The listing builds one solid part. Answer for the finished solid, in the listing's coordinates (mm). Round coordinates to 2 decimals unless told otherwise and drop trailing zeros. Write each loop counter-clockwise with the first axis right and the second up, starting at its lowest first coordinate (ties: lowest second). Pieces come first, ordered by that corner, then holes. Notation, with made-up numbers: (79, 47.5) - (85, 47.5) arc R32 ccw to (85, 75.5) - close; hole circle Ø4 at (38.5, 44). An arc over 180 degrees is marked (long way). Use a Markdown table: item, result. Add a question column.
1) A cutting plane is placed at A-A (z = 74.5). Give the vertices of the cut face in (x, y).
2) Find the intervals of material crossed by probe 1 along Z at (x, y) = (0, 2.1); probe 2 along Z at (x, y) = (60, 2.2); probe 3 along X at (y, z) = (2.15, 72), in increasing order. Write a range as from..to.
3) Each of these flat-tipped pins is pushed along its axis until it touches: P1, Ø0.9, axis at y = 1.5, z = 78, coming from the -X side; P2, Ø1.5, axis at x = 0, y = 1.5, coming from the -Z side; P3, Ø1.8, axis at x = 75, z = -60, coming from the -Y side. Where does it stop, or does it pass through?
4) A cutting plane is placed at C-C (z = 44). Give the vertices of the cut face in (x, y), then the cut area to 3 significant figures.
5) A cutting plane is placed at B-B (y = 0.95). State how many separate pieces and enclosed holes the cut face has, then the cut area to 3 significant figures.
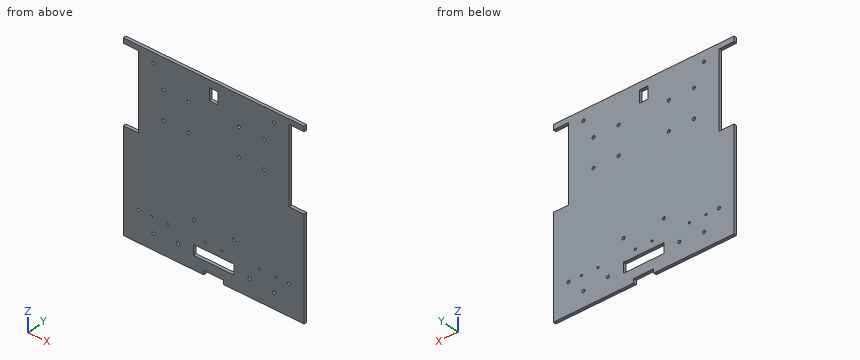
```python
from build123d import *

# Parameters (mm, degrees)
SKETCH1_W           = 180
SKETCH1_H           = 180
BOSS_EXTRUDE1_DEPTH = 3
SKETCH2_W           = 15
SKETCH2_H           = 75
CUT_EXTRUDE1_DEPTH  = 3
SKETCH3_R           = 1.5
SKETCH3_R_2         = 1
SKETCH3_W           = 40
SKETCH3_H           = 10
CUT_EXTRUDE2_DEPTH  = 3
SKETCH5_R           = 1.5
CUT_EXTRUDE3_DEPTH  = 3
SKETCH7_W           = 20
SKETCH7_H           = 4
CUT_EXTRUDE4_DEPTH  = 3
SKETCH8_W           = 8.5
SKETCH8_H           = 12
CUT_EXTRUDE5_DEPTH  = 3


with BuildPart() as part:
    # Sketch1 → Boss-Extrude1 (new body)
    with BuildSketch(Plane(origin=(0, 0, 0), x_dir=(1, 0, 0), z_dir=(0, 1, 0))):
        Rectangle(SKETCH1_W, SKETCH1_H)
    extrude(amount=BOSS_EXTRUDE1_DEPTH)

    # Sketch2 → Cut-Extrude1 (cut)
    with BuildSketch(Plane(origin=(0, 3, 0), x_dir=(1, 0, 0), z_dir=(0, 1, 0))):
        with Locations((-82.5, -47.5)):
            Rectangle(SKETCH2_W, SKETCH2_H)
        with Locations((82.5, -47.5)):
            Rectangle(SKETCH2_W, SKETCH2_H)
    extrude(amount=-CUT_EXTRUDE1_DEPTH, mode=Mode.SUBTRACT)

    # Sketch3 → Cut-Extrude2 (cut)
    with BuildSketch(Plane(origin=(0, 3, 0), x_dir=(1, 0, 0), z_dir=(0, 1, 0))):
        with Locations(Location((-50, -32.5, 0), (0, 0, 270))):
            Circle(SKETCH3_R)
        with Locations(Location((-50, -60.5, 0), (0, 0, 270))):
            Circle(SKETCH3_R)
        with Locations(Location((-25, -32.5, 0), (0, 0, 270))):
            Circle(SKETCH3_R)
        with Locations(Location((-25, -60.5, 0), (0, 0, 270))):
            Circle(SKETCH3_R)
        with Locations(Location((25, -60.5, 0), (0, 0, 90))):
            Circle(SKETCH3_R)
        with Locations(Location((50, -60.5, 0), (0, 0, 90))):
            Circle(SKETCH3_R)
        with Locations(Location((25, -32.5, 0), (0, 0, 90))):
            Circle(SKETCH3_R)
        with Locations(Location((50, -32.5, 0), (0, 0, 90))):
            Circle(SKETCH3_R)
        with Locations(Location((-60, -80, 0), (0, 0, 270))):
            Circle(SKETCH3_R)
        with Locations(Location((60, -80, 0), (0, 0, 90))):
            Circle(SKETCH3_R)
        with Locations(Location((-62, 60, 0), (0, 0, 270))):
            Circle(SKETCH3_R_2)
        with Locations(Location((-45.5, 60, 0), (0, 0, 270))):
            Circle(SKETCH3_R_2)
        with Locations(Location((45.5, 60, 0), (0, 0, 90))):
            Circle(SKETCH3_R_2)
        with Locations(Location((62, 60, 0), (0, 0, 90))):
            Circle(SKETCH3_R_2)
        with Locations(Location((-60, 75, 0), (0, 0, 270))):
            Circle(SKETCH3_R)
        with Locations(Location((60, 75, 0), (0, 0, 90))):
            Circle(SKETCH3_R)
        with Locations(Location((-8.25, 60, 0), (0, 0, 270))):
            Circle(SKETCH3_R_2)
        with Locations(Location((8.25, 60, 0), (0, 0, 90))):
            Circle(SKETCH3_R_2)
        with Locations(Location((-20, 44.727497325, 0), (0, 0, 270))):
            Circle(SKETCH3_R)
        with Locations(Location((20, 44.727497325, 0), (0, 0, 90))):
            Circle(SKETCH3_R)
        with Locations((0, 71.727497325)):
            Rectangle(SKETCH3_W, SKETCH3_H)
    extrude(amount=-CUT_EXTRUDE2_DEPTH, mode=Mode.SUBTRACT)

    # Sketch5 → Cut-Extrude3 (cut)
    with BuildSketch(Plane(origin=(0, 3, 0), x_dir=(1, 0, 0), z_dir=(0, 1, 0))):
        with Locations(Location((-75, 60, 0), (0, 0, 270))):
            Circle(SKETCH5_R)
        with Locations(Location((75, 60, 0), (0, 0, 90))):
            Circle(SKETCH5_R)
        with Locations(Location((-35.5, 73, 0), (0, 0, 270))):
            Circle(SKETCH5_R)
        with Locations(Location((35.5, 73, 0), (0, 0, 90))):
            Circle(SKETCH5_R)
    extrude(amount=-CUT_EXTRUDE3_DEPTH, mode=Mode.SUBTRACT)

    # Sketch7 → Cut-Extrude4 (cut)
    with BuildSketch(Plane(origin=(0, 3, 0), x_dir=(1, 0, 0), z_dir=(0, 1, 0))):
        with Locations((0, 88)):
            Rectangle(SKETCH7_W, SKETCH7_H)
    extrude(amount=-CUT_EXTRUDE4_DEPTH, mode=Mode.SUBTRACT)

    # Sketch8 → Cut-Extrude5 (cut)
    with BuildSketch(Plane(origin=(0, 3, 0), x_dir=(1, 0, 0), z_dir=(0, 1, 0))):
        with Locations((0, -77)):
            Rectangle(SKETCH8_W, SKETCH8_H)
    extrude(amount=-CUT_EXTRUDE5_DEPTH, mode=Mode.SUBTRACT)


solid = part.part
```
Entries:
| question | item | result |
|---|---|---|
| 1 | outline | (-75, 0) - (-4.25, 0) - (-4.25, 3) - (-75, 3) - close; (4.25, 0) - (75, 0) - (75, 3) - (4.25, 3) - close |
| 2 | probe 1 | z = -86..-76.73, -66.73..71, 83..90 |
| 2 | probe 2 | z = -90..-76.5, -73.5..78.5, 81.5..90 |
| 2 | probe 3 | x = -75..-4.25, 4.25..75 |
| 3 | P1 | stops at x = -75 |
| 3 | P2 | stops at z = -86 |
| 3 | P3 | passes through |
| 4 | outline | (-75, 0) - (75, 0) - (75, 3) - (-75, 3) - close |
| 4 | area | 450 mm² |
| 5 | separate pieces | 1 |
| 5 | enclosed holes | 26 |
| 5 | area | 29,400 mm² |
